The drawing under review shows one solid part. Ordinate dimensions are in mm from its lowest x, y, z. A direction names the side the tool comes from. Coordinates: 2 decimals unless noted, no trailing zeros. Loops run counter-clockwise (first coordinate to the right, second up) from the corner with the lowest first, then second, coordinate; pieces in that order, holes last.
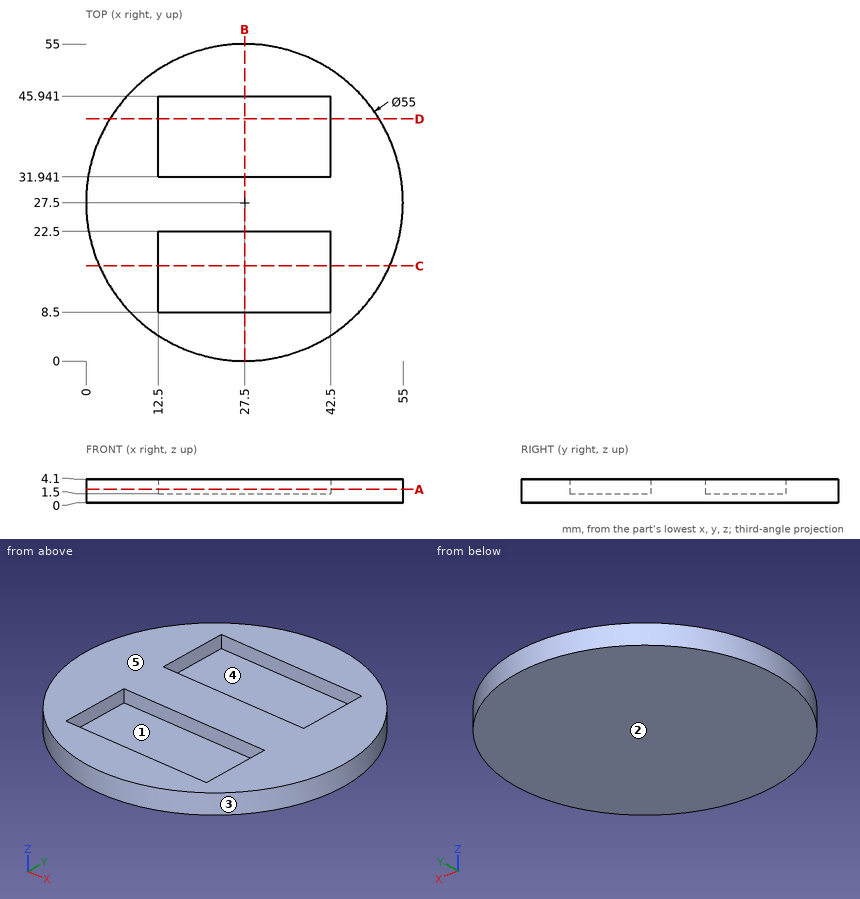
Q1. Take a section at D-D, the plane y = 42. Write out the cut boundary in (x, z).
Q2. Take a section at B-B, the plane x = 27.5. Write out the cut boundary in (y, z), then the cut area to 3 significant figures.
Q3. Clearance check with flat-ended pins moving along their axes: pin 1 Ø1.3 at (x, z) = (30.5, 2.5) entering from +Y; pin 2 Ø1.3 at (y, z) = (12.5, 3) entering from +X; pin 3 Ø1.3 at (x, z) = (32, 2.5) entering from +Y; pin 4 Ø6 at (x, y) = (18.5, 22) entering from +Z. State where each tip first meets the part, or that it passes through.
Q4. Take a section at A-A, the plane z = 2.3. Write out the cut boundary in (x, y), then the cut area to 3 significant figures.
Q5. The part is to be moulded in two halves that separate along X. For the marked faces 3, 4 and 5, say which applies: pulls with the +X half, pulls with the -X half, needs draft (parallel to the pull), parting line crosses it, or undercut.
Q6. Machinability: for the marked faces 1 and 2, which of the approach directions +Z, -Z, +X, -X, +Y, -Y give a long, thin tool a straight path to every point of the face, cutting with its end or side? Answer none if there is none.
Q7. For line 1 (Y direction, x = 40.5, z = 2.25); line 2 (Y direction, x = 39, z = 3.4); line 3 (X direction, y = 18, z = 3.7), list the stretches that pass through material, from the lowest coordinate up.
Q8. Take a section at C-C, the plane y = 16.5. Write out the cut boundary in (x, z), then the cut area to 3 significant figures.
Entries:
1. outline: (4.13, 0) - (50.87, 0) - (50.87, 4.1) - (42.5, 4.1) - (42.5, 1.5) - (12.5, 1.5) - (12.5, 4.1) - (4.13, 4.1) - close
2. outline: (0, 0) - (55, 0) - (55, 4.1) - (45.94, 4.1) - (45.94, 1.5) - (31.94, 1.5) - (31.94, 4.1) - (22.5, 4.1) - (22.5, 1.5) - (8.5, 1.5) - (8.5, 4.1) - (0, 4.1) - close
2. area: 153 mm2
3. pin 1: stops at y = 54.9
3. pin 2: stops at x = 50.96
3. pin 3: stops at y = 54.73
3. pin 4: stops at z = 4.1
4. outline: circle Ø55 at (27.5, 27.5); hole (12.5, 8.5) - (42.5, 8.5) - (42.5, 22.5) - (12.5, 22.5) - close; hole (12.5, 31.94) - (42.5, 31.94) - (42.5, 45.94) - (12.5, 45.94) - close
4. area: 1,540 mm2
5. face 3: parting line crosses it
5. face 4: undercut
5. face 5: needs draft
6. face 1: +Z
6. face 2: -Z, +X, -X, +Y, -Y
7. line 1: y = 3.27 to 8.5, 22.5 to 31.94, 45.94 to 51.73
7. line 2: y = 2.52 to 8.5, 22.5 to 31.94, 45.94 to 52.48
7. line 3: x = 1.69 to 12.5, 42.5 to 53.31
8. outline: (2.3, 0) - (52.7, 0) - (52.7, 4.1) - (42.5, 4.1) - (42.5, 1.5) - (12.5, 1.5) - (12.5, 4.1) - (2.3, 4.1) - close
8. area: 129 mm2
